Model file for the job. Use its own axes, mm. A direction names the side the tool comes from. Round coordinates to 2 decimals unless told otherwise and drop trailing zeros. Order: outer loops, then holes, each group sorted by start corner. A loop starts at its lowest first (then second) coordinate and runs counter-clockwise, first axis right, second up. Notation, with made-up numbers: (34, -37) - (70, -37) arc R35 cw to (70, -5) - close; hole circle Ø10 at (76.25, 54.25). An arc over 180 degrees is marked (long way). Answer as CSV lines item,"result". Start each with the question number.
1. Band-saw the part on B-B on x = 0. List the corners of the cut face in (y, z), then the cut area to 3 significant figures.
2. Pin check, flat tips, straight feed: pin 1 Ø3 at (x, z) = (-17.5, -48.5) entering from -Y; pin 2 Ø5 at (y, z) = (18, -139.5) entering from +X; pin 3 Ø8 at (y, z) = (-4.5, 0) entering from -X. Stop position of each tip, or through.
3. Band-saw the part on A-A on y = 0. List the corners of the cut face in (x, z).
4. 3-axis set-ups, long thin cutter, end or side, ignore diameter. For faces 3 (the face through (-3.78, 17.04, -104.07)), 4 (the face through (-14.247, -64.158, -14.277)): which of +Z, -Z, +X, -X, +Y, -Y reach the whole face in a straight line?
5. Wall check: line 1 along Z through (x, y) = (10, 33); line 2 along X through (y, z) = (-5, 19); line 3 along X through (y, z) = (-3.5, -168). Give the ranges that are in metal, low to high. Write a range as [from, to].
6. Band-saw the part on C-C on z = -86.5. List the corners of the cut face in (x, y), then the cut area to 3 significant figures.
7. Pull direction Y, two halves, no side cores. Call faces 1 (the face through (43.536, 1.935, 25.814)), 2 (the face through (-1, 1, 0)): released by +Y, released by -Y, zero draft, split by the parting line, or undercut.
8. Band-saw the part on D-D on z = 17. List the corners of the cut face in (x, y), then the cut area to 3 significant figures.
```python
from build123d import *

# Parameters (mm, degrees)
F0_R     = 65.720359
F1_DEPTH = 28.95929
F2_R     = 6.440995
F3_DEPTH = 52.36186
F4_R     = 17.45325
F5_DEPTH = 152.35555


with BuildPart() as f1:
    # F0 (on Top) → F1 (new body)
    with BuildSketch(Plane.XY):
        Circle(F0_R)
    extrude(amount=-F1_DEPTH)

    # F2 (on Top) → F3 (join)
    with BuildSketch(Plane.XY):
        with Locations((37.392426, 0)):
            Circle(F2_R)
    extrude(amount=F3_DEPTH)

    # F4 (on face) → F5 (join)
    with BuildSketch(Plane(origin=(0, 0, -28.95929), x_dir=(1, 0, 0), z_dir=(0, 0, -1))):
        Circle(F4_R)
    extrude(amount=F5_DEPTH)


solid = f1.part
```
Reply:
1,outline,"(-65.72, -28.96) - (-17.45, -28.96) - (-17.45, -181.31) - (17.45, -181.31) - (17.45, -28.96) - (65.72, -28.96) - (65.72, 0) - (-65.72, 0) - close"
1,area,"9,120 mm2"
2,pin 1,"stops at y = -6.97"
2,pin 2,"stops at x = 8.02"
2,pin 3,"stops at x = -65.72"
3,outline,"(-65.72, -28.96) - (-17.45, -28.96) - (-17.45, -181.31) - (17.45, -181.31) - (17.45, -28.96) - (65.72, -28.96) - (65.72, 0) - (43.83, 0) - (43.83, 52.36) - (30.95, 52.36) - (30.95, 0) - (-65.72, 0) - close"
4,face 3,"-Z"
4,face 4,"+Z, -Z"
5,line 1,"z = [-28.96, 0]"
5,line 2,"x = [33.33, 41.45]"
5,line 3,"x = [-17.1, 17.1]"
6,outline,"circle Ø34.91 at (0, 0)"
6,area,"957 mm2"
7,face 1,"split by the parting line"
7,face 2,"zero draft"
8,outline,"circle Ø12.88 at (37.39, 0)"
8,area,"130 mm2"
